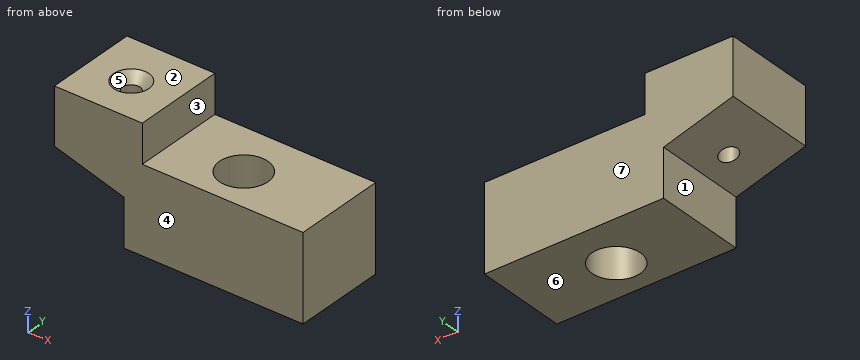
from build123d import *

# Parameters (mm, degrees)
F1_DEPTH       = 29.21
F2_R           = 7.6633678856
F3_DEPTH       = 41.402
F5_D           = 5.5
F5_CSINK_D     = 11.2
F5_CSINK_ANGLE = 90


with BuildPart() as f1:
    # F0 (on Front) → F1 (new body)
    with BuildSketch(Plane.XZ):
        Polygon((-42.0007146895, 25.8535724133), (-42.0007146895, 8.0735711381), (-20.0478583574, 1.7235714477), (-20.0478583574, -13.3350007236), (36.5578569472, -13.3350007236), (36.5578569472, 13.6978570372), (-14.2421433702, 13.6978570372), (-14.2421433702, 25.8535724133), align=None)
    extrude(amount=F1_DEPTH)

    # F2 (on face) → F3 (cut)
    with BuildSketch(Plane.XY.offset(13.6978570372)):
        with Locations((7.6602338813, -16.2490848452)):
            Circle(F2_R)
    extrude(amount=-F3_DEPTH, mode=Mode.SUBTRACT)

    # F5 (through all)
    with Locations(Plane.XY.offset(25.8535724133)):
        with Locations((-28.3485297114, -15.6557932496)):
            CounterSinkHole(F5_D / 2, F5_CSINK_D / 2, counter_sink_angle=F5_CSINK_ANGLE)


solid = f1.part
Input: part model. Units: mm. Frame: model coordinates. Face numbers are marked on the shaded views. A direction names the side the tool comes from. Coordinates: 2 decimals unless noted, no trailing zeros. Order: outer loops, then holes, each group sorted by start corner. A loop starts at its lowest first (then second) coordinate and runs counter-clockwise, first axis right, second up.
1. Access query for the marked faces 1, 2 and 3. Directions: +Z, -Z, +X, -X, +Y, -Y. A direction counts if a zero-diameter tool reaches every point of the face in a straight line with its end or side. Return the directions, or none.
Checked values:
face 1: -Z, -X, +Y, -Y
face 2: +Z, +X, -X, +Y, -Y
face 3: +Z, +X, +Y, -Y
2. Cut plane B-B, the plane x = 6. Return loops of the section in (y, z) (3 decimals), plus the area to 3 significant figures.
Checked values:
outline: (-29.21, -13.335) - (-23.73, -13.335) - (-23.73, 13.698) - (-29.21, 13.698) - close; (-8.768, -13.335) - (0, -13.335) - (0, 13.698) - (-8.768, 13.698) - close
area: 385 mm2
3. Cut plane D-D, the plane z = 12.5. Return loops of the section in (x, y), plus the area to 3 significant figures.
Checked values:
outline: (-42, -29.21) - (36.56, -29.21) - (36.56, 0) - (-42, 0) - close; hole circle Ø5.5 at (-28.35, -15.66); hole circle Ø15.33 at (7.66, -16.25)
area: 2,090 mm2
4. Contact query for flat-ended pins moving along their axis: P1, Ø2, axis at x = 10, y = -23, coming from the -Z side (3 decimals); P2, Ø6, axis at x = 5.5, y = -23, coming from the +Z side; P3, Ø6.5, axis at x = -28.35, y = -15.66, coming from the +Z side; P4, Ø12, axis at y = -8, z = -5, coming from the -X side. Output: stop coordinate, or through.
Checked values:
P1: stops at z = -13.335
P2: stops at z = 13.7
P3: stops at z = 23.51
P4: stops at x = -20.05
5. Cut plane C-C, the plane z = -10. Return loops of the section in (x, y).
Checked values:
outline: (-20.05, -29.21) - (36.56, -29.21) - (36.56, 0) - (-20.05, 0) - close; hole circle Ø15.33 at (7.66, -16.25)
6. Draft query along Y for the marked faces 4, 5, 6 and 7. Return one class per face: +Y half, -Y half, draft (parallel to the pull), parting line (faces both ways), or undercut.
Checked values:
face 4: -Y half
face 5: undercut
face 6: draft
face 7: +Y half
7. Cut plane A-A, the plane y = -26.75. Return loops of the section in (x, z) (3 decimals).
Checked values:
outline: (-42.001, 8.074) - (-20.048, 1.724) - (-20.048, -13.335) - (36.558, -13.335) - (36.558, 13.698) - (-14.242, 13.698) - (-14.242, 25.854) - (-42.001, 25.854) - close
8. Ray query, line 1 along X through (y, z) = (-16.25, -8.5); line 2 along Z through (x, y) = (-9, -8.5) (3 decimals); line 3 along X through (y, z) = (-5.25, -4.5). Return the intervals inside material, ascending.
Checked values:
line 1: x = -20.05 to 0, 15.32 to 36.56
line 2: z = -13.335 to 13.698
line 3: x = -20.05 to 36.56
